Can you work these out from the model? Positions are in its coordinate system, mm. A direction names the side the tool comes from. Round coordinates to 2 decimals unless told otherwise and drop trailing zeros. Loops run counter-clockwise (first coordinate to the right, second up) from the corner with the lowest first, then second, coordinate; pieces in that order, holes last.
(1) Will these pins go through, and if not, where does the flat tip stop? pin 1 Ø6.5 at (x, y) = (-20.5, -59) entering from +Z; pin 2 Ø3 at (x, y) = (0.5, -29.5) entering from +Z; pin 3 Ø2.5 at (x, y) = (-19.05, -57.66) entering from +Z; pin 4 Ø2.5 at (x, y) = (-18.5, -9.5) entering from +Z.
(2) I want a section at C-C on x = 0. Write out the boundary of the cut face in (y, z) (3 decimals), plus the area to 3 significant figures.
(3) Thinking about a two-plate mould opening in X: for faces 1 (the face through (0, -67.66, -9)), 2 (the face through (-18, -10, -12.5)), 3 (the face through (26, -33, -9)), which applies, released by +X, released by -X, zero draft, split by the parting line, or undercut?
(4) I want a section at D-D on y = -10. Write out the boundary of the cut face in (x, z) (3 decimals), plus the area to 3 significant figures.
(5) I want a section at A-A on z = -7. Write out the boundary of the cut face in (x, y) (3 decimals), plus the area to 3 significant figures.
(6) I want a section at B-B on y = -30. Write out the boundary of the cut face in (x, z) (3 decimals), plus the area to 3 significant figures.
(7) Which directions (+Z, -Z, +X, -X, +Y, -Y) give clear straight access to the entire face, cutting with the end or side of a thin tool? Please do faces 4 (the face through (0, -34, -17.5)), 5 (the face through (19.18, -12.26, -6.16)).
(8) If I drill on line 1 along Y through (x, z) = (0, -3.5) (3 decimals); line 2 along Y through (x, z) = (19.05, -14.5) (3 decimals); line 3 along X through (y, z) = (-30, -15.2) (3 decimals), over which ranges is the centre line in solid material (lowest first)?
from build123d import *

# Parameters (mm, degrees)
F1_W     = 52
F1_H     = 67.66
F2_DEPTH = 17.5
F0_R     = 1.575
F3_DEPTH = 17.5
F4_R     = 2.875
F5_DEPTH = 13.5
F6_R     = 2.55
F7_DEPTH = 12.5
F8_ANGLE = 180
F9_ANGLE = 180


with BuildPart() as f2:
    # F1 (on Top) → F2 (new body)
    with BuildSketch(Plane.XY):
        with Locations((0, 3.83)):
            Rectangle(F1_W, F1_H)
    extrude(amount=F2_DEPTH)

    # F0 (on Top) → F3 (cut)
    with BuildSketch(Plane.XY):
        Circle(F0_R)
        with Locations((0, -20)):
            Circle(F0_R)
        with Locations((-19.05, 27.66)):
            Circle(F0_R)
        with Locations((19.05, 27.66)):
            Circle(F0_R)
    extrude(amount=F3_DEPTH, mode=Mode.SUBTRACT)

    # F4 (on face) → F5 (cut)
    with BuildSketch(Plane(origin=(0, 0, 0), x_dir=(1, 0, 0), z_dir=(0, 0, -1))):
        Circle(F4_R)
        with Locations((19.05, -27.66)):
            Circle(F4_R)
        with Locations((-19.05, -27.66)):
            Circle(F4_R)
        with Locations((0, 20)):
            Circle(F4_R)
    extrude(amount=-F5_DEPTH, mode=Mode.SUBTRACT)

    # F6 (on face) → F7 (cut)
    with BuildSketch(Plane(origin=(0, 0, 0), x_dir=(1, 0, 0), z_dir=(0, 0, -1))):
        with Locations((0, -28)):
            Circle(F6_R)
        with Locations((-18, 20)):
            Circle(F6_R)
        with Locations((18, 20)):
            Circle(F6_R)
    extrude(amount=-F7_DEPTH, mode=Mode.SUBTRACT)


with BuildPart() as f2_1:
    # F8: moved
    add(f2.part.rotate(Axis((-26, 3.83, 17.5), (0, 1, 0)), F8_ANGLE))


with BuildPart() as f2_2:
    # F9: moved
    add(f2_1.part.rotate(Axis((-26, 37.66, 26.25), (0, 0, 1)), F9_ANGLE))


with BuildPart() as f2_3:
    # F11: moved
    add(f2_2.part.moved(Location((0, -105.32, -35))))


solid = f2_3.part
Filled sheet:
1. pin 1: stops at z = 0
1. pin 2: stops at z = -13.5
1. pin 3: passes through
1. pin 4: stops at z = -12.5
2. outline: (-67.66, -17.5) - (-31.575, -17.5) - (-31.575, -13.5) - (-32.875, -13.5) - (-32.875, 0) - (-55.45, 0) - (-55.45, -12.5) - (-60.55, -12.5) - (-60.55, 0) - (-67.66, 0) - close; (-28.425, -17.5) - (-11.575, -17.5) - (-11.575, -13.5) - (-12.875, -13.5) - (-12.875, 0) - (-27.125, 0) - (-27.125, -13.5) - (-28.425, -13.5) - close; (-8.425, -17.5) - (0, -17.5) - (0, 0) - (-7.125, 0) - (-7.125, -13.5) - (-8.425, -13.5) - close
2. area: 940 mm2
3. face 1: zero draft
3. face 2: undercut
3. face 3: released by +X
4. outline: (-26, -17.5) - (-1.575, -17.5) - (-1.575, -13.5) - (-2.875, -13.5) - (-2.875, 0) - (-15.45, 0) - (-15.45, -12.5) - (-20.55, -12.5) - (-20.55, 0) - (-26, 0) - close; (1.575, -17.5) - (26, -17.5) - (26, 0) - (20.55, 0) - (20.55, -12.5) - (15.45, -12.5) - (15.45, 0) - (2.875, 0) - (2.875, -13.5) - (1.575, -13.5) - close
4. area: 692 mm2
5. outline: (-26, -67.66) - (26, -67.66) - (26, 0) - (-26, 0) - close; hole circle Ø5.75 at (-19.05, -57.66); hole circle Ø5.1 at (-18, -10); hole circle Ø5.75 at (0, -30); hole circle Ø5.75 at (0, -10); hole circle Ø5.1 at (0, -58); hole circle Ø5.1 at (18, -10); hole circle Ø5.75 at (19.05, -57.66)
5. area: 3,350 mm2
6. outline: (-26, -17.5) - (-1.575, -17.5) - (-1.575, -13.5) - (-2.875, -13.5) - (-2.875, 0) - (-26, 0) - close; (1.575, -17.5) - (26, -17.5) - (26, 0) - (2.875, 0) - (2.875, -13.5) - (1.575, -13.5) - close
6. area: 820 mm2
7. face 4: -Z, +X, -X, +Y, -Y
7. face 5: +Z
8. line 1: y = -67.66 to -60.55, -55.45 to -32.875, -27.125 to -12.875, -7.125 to 0
8. line 2: y = -67.66 to -59.235, -56.085 to 0
8. line 3: x = -26 to -1.575, 1.575 to 26
